Geometry check sheet. Reference: the model listing, model coordinates, mm. Coordinates: 2 decimals unless noted, no trailing zeros. Write each loop counter-clockwise with the first axis right and the second up, starting at its lowest first coordinate (ties: lowest second). Pieces come first, ordered by that corner, then holes. Notation, with made-up numbers: (76, 32) -> (117, 32) arc R21 cw to (117, 42) -> close; hole circle Ø7 at (-17, -12.75). An arc over 180 degrees is marked (long way). Answer in a Markdown table with one row per item. Add a question column.
1. Cross-section at D-D on z = -213. Record the cut outline in (x, y).
2. Scan lines: L1, parallel to X at y = 0.9, z = 0; L2, parallel to Z at x = -25, y = 1.3; L3, parallel to Z at x = -50, y = 1.95. Record each from-to range of solid material in increasing order. Write a range as from..to.
3. Depth check by flat-ended pin: P1, Ø1.5, axis at x = -75.5, y = 0.5, coming from the +Z side; P2, Ø1, axis at x = 191.5, y = 0.5, coming from the -Z side. Enter the tip coordinate at first touch or a pass-through.
4. Cross-section at A-A on x = 0. Record the cut outline in (y, z).
5. Cross-section at C-C on x = 145. Record the cut outline in (y, z), and give its area (3 significant figures).
6. Mould release check, pull along Z, two halves, no side actions. Record for faces 1 (the flat face through (-5, 0, 78)), 2 (the cylindrical face through (-15.12, 1.57, 11.59)), 3 (the cylindrical face through (201.6, 1.5, -316.2)): pulls with the +Z half, pulls with the -Z half, needs draft (parallel to the pull), parting line crosses it, or undercut.
7. Cross-section at B-B on y = 1.75. Give the number of separate pieces and of enclosed holes in the cut face, and give its area (3 significant figures).
```python
from build123d import *

# Parameters (mm, degrees)
CROQUIS1_R              = 375
SALIENTE_EXTRUIR1_DEPTH = 3.1
CROQUIS3_R              = 6.35
CROQUIS3_R_2            = 19.05
CORTAR_EXTRUIR2_DEPTH   = 4.1
CROQUIS4_R              = 4
CORTAR_EXTRUIR3_DEPTH   = 4.1


with BuildPart() as part:
    # Croquis1 → Saliente-Extruir1 (new body)
    with BuildSketch(Plane(origin=(0, 0, 0), x_dir=(1, 0, 0), z_dir=(0, 1, 0))):
        Circle(CROQUIS1_R)
    extrude(amount=SALIENTE_EXTRUIR1_DEPTH)

    # Croquis3 → Cortar-Extruir2 (cut, through all)
    with BuildSketch(Plane(origin=(0, 3.1, 0), x_dir=(1, 0, 0), z_dir=(0, 1, 0))):
        with Locations((-251.871435459, -251.871435459)):
            Circle(CROQUIS3_R)
        with Locations((-251.871435459, 251.871435459)):
            Circle(CROQUIS3_R)
        with Locations((251.871435459, 251.871435459)):
            Circle(CROQUIS3_R)
        with Locations((251.871435459, -251.871435459)):
            Circle(CROQUIS3_R)
        Circle(CROQUIS3_R_2)
    extrude(amount=-CORTAR_EXTRUIR2_DEPTH, mode=Mode.SUBTRACT)

    # Croquis4 → Cortar-Extruir3 (cut, through all)
    with BuildSketch(Plane(origin=(0, 3.1, 0), x_dir=(1, 0, 0), z_dir=(0, 1, 0))):
        with Locations((50, 0)):
            Circle(CROQUIS4_R)
        with Locations((25, -43.301270189)):
            Circle(CROQUIS4_R)
        with Locations((-25, -43.301270189)):
            Circle(CROQUIS4_R)
        with Locations((-50, 0)):
            Circle(CROQUIS4_R)
        with Locations((-25, 43.301270189)):
            Circle(CROQUIS4_R)
        with Locations((25, 43.301270189)):
            Circle(CROQUIS4_R)
    extrude(amount=-CORTAR_EXTRUIR3_DEPTH, mode=Mode.SUBTRACT)


solid = part.part
```
Results found:
| question | item | result |
|---|---|---|
| 1 | outline | (-308.64, 0) -> (308.64, 0) -> (308.64, 3.1) -> (-308.64, 3.1) -> close |
| 2 | L1 | x = -375..-54, -46..-19.05, 19.05..46, 54..375 |
| 2 | L2 | z = -374.17..-47.3, -39.3..39.3, 47.3..374.17 |
| 2 | L3 | z = -371.65..-4, 4..371.65 |
| 3 | P1 | stops at z = 367.47 |
| 3 | P2 | stops at z = -322.71 |
| 4 | outline | (0, -375) -> (3.1, -375) -> (3.1, -19.05) -> (0, -19.05) -> close; (0, 19.05) -> (3.1, 19.05) -> (3.1, 375) -> (0, 375) -> close |
| 5 | outline | (0, -345.83) -> (3.1, -345.83) -> (3.1, 345.83) -> (0, 345.83) -> close |
| 5 | area | 2,140 mm^2 |
| 6 | face 1 | needs draft |
| 6 | face 2 | undercut |
| 6 | face 3 | parting line crosses it |
| 7 | separate pieces | 1 |
| 7 | enclosed holes | 11 |
| 7 | area | 440,000 mm^2 |
